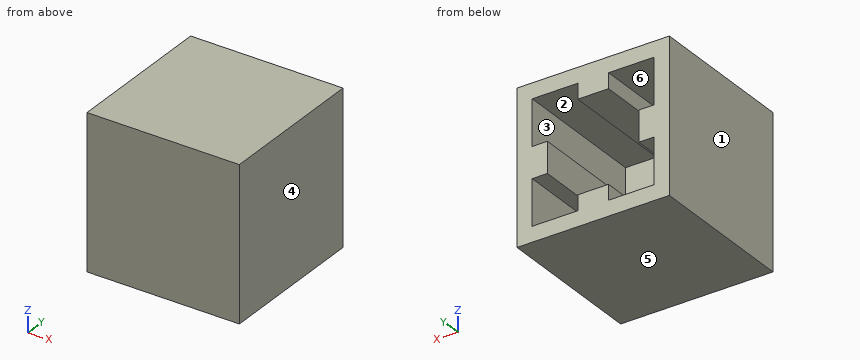
from build123d import *

# Parameters (mm, degrees)
SKETCH1_W           = 25.4
SKETCH1_H           = 25.4
BOSS_EXTRUDE1_DEPTH = 25.4
CUT_EXTRUDE2_DEPTH  = 22.86


with BuildPart() as part:
    # Sketch1 → Boss-Extrude1 (new body)
    with BuildSketch(Plane(origin=(0, 0, 0), x_dir=(1, 0, 0), z_dir=(0, 1, 0))):
        Rectangle(SKETCH1_W, SKETCH1_H)
    extrude(amount=BOSS_EXTRUDE1_DEPTH)

    # Sketch3 → Cut-Extrude2 (cut)
    with BuildSketch(Plane(origin=(0, 25.4, 0), x_dir=(1, 0, 0), z_dir=(0, 1, 0))):
        Polygon((10.16, 2.565122784), (7.62, 2.565122784), (7.62, -2.565122784), (10.16, -2.565122784), (10.16, -10.16), (2.565122784, -10.16), (2.565122784, -7.62), (-2.565122784, -7.62), (-2.565122784, -10.16), (-10.16, -10.16), (-10.16, -2.565122784), (-7.62, -2.565122784), (-7.62, 2.565122784), (-10.16, 2.565122784), (-10.16, 10.16), (-2.565122784, 10.16), (-2.565122784, 7.62), (2.565122784, 7.62), (2.565122784, 10.16), (10.16, 10.16), align=None)
    extrude(amount=-CUT_EXTRUDE2_DEPTH, mode=Mode.SUBTRACT)


solid = part.part
Design review of the part built by this model. Coordinates are the model's own, in mm. Face numbers are marked on the shaded views. A direction names the side the tool comes from. Give positions to 0.01 mm unless a question says otherwise; leave off trailing zeros. Order: outer loops, then holes, each group sorted by start corner. A loop starts at its lowest first (then second) coordinate and runs counter-clockwise, first axis right, second up. Notation, with made-up numbers: (64, 85) - (114, 85) arc R12 cw to (114, 103) - close; hole circle Ø2 at (69, 58.25). An arc over 180 degrees is marked (long way). Use CSV: the item, a comma, the result in double quotes. Start each with the question number.
Q1. Machinability: for the marked faces 1 and 2, which of the approach directions +Z, -Z, +X, -X, +Y, -Y give a long, thin tool a straight path to every point of the face, cutting with its end or side? Answer none if there is none.
Q2. Take a section at A-A (y = 16.5). State the section outline as (x, z) points.
Q3. For P1, Ø1, axis at x = 8, z = 6, coming from the +Y side, flat-tipped, find the tip position at first contact; note if it passes through.
Q4. Take a section at C-C (x = -6.75). State the section outline as (y, z) points, and give its area (3 significant figures).
Q5. Take a section at B-B (z = 6.5). State the section outline as (x, y) points, and give its area (3 significant figures).
Q6. Draft analysis for pull direction Z (two halves, no side actions). For the marked faces 3, 4, 5 and 6, state which applies: pulls with the +Z half, pulls with the -Z half, needs draft (parallel to the pull), parting line crosses it, or undercut.
Q7. For line 1 (X direction, y = 12.25, z = 9.5); line 2 (X direction, y = 23.5, z = -2.25), list the stretches that pass through material, from the lowest coordinate up.
Calculated:
1,face 1,"+Z, -Z, -X, +Y, -Y"
1,face 2,"+Y"
2,outline,"(-12.7, -12.7) - (12.7, -12.7) - (12.7, 12.7) - (-12.7, 12.7) - close; hole (-10.16, -10.16) - (-2.57, -10.16) - (-2.57, -7.62) - (2.57, -7.62) - (2.57, -10.16) - (10.16, -10.16) - (10.16, -2.57) - (7.62, -2.57) - (7.62, 2.57) - (10.16, 2.57) - (10.16, 10.16) - (2.57, 10.16) - (2.57, 7.62) - (-2.57, 7.62) - (-2.57, 10.16) - (-10.16, 10.16) - (-10.16, 2.57) - (-7.62, 2.57) - (-7.62, -2.57) - (-10.16, -2.57) - close"
3,P1,"stops at y = 2.54"
4,outline,"(0, -12.7) - (25.4, -12.7) - (25.4, -10.16) - (2.54, -10.16) - (2.54, 10.16) - (25.4, 10.16) - (25.4, 12.7) - (0, 12.7) - close"
4,area,"181 mm²"
5,outline,"(-12.7, 0) - (12.7, 0) - (12.7, 25.4) - (10.16, 25.4) - (10.16, 2.54) - (-10.16, 2.54) - (-10.16, 25.4) - (-12.7, 25.4) - close"
5,area,"181 mm²"
6,face 3,"undercut"
6,face 4,"needs draft"
6,face 5,"pulls with the -Z half"
6,face 6,"undercut"
7,line 1,"x = -12.7 to -10.16, -2.57 to 2.57, 10.16 to 12.7"
7,line 2,"x = -12.7 to -7.62, 7.62 to 12.7"
